Design review of the part built by this model. Coordinates are the model's own, in mm. A direction names the side the tool comes from. Coordinates: 2 decimals unless noted, no trailing zeros. Loops run counter-clockwise (first coordinate to the right, second up) from the corner with the lowest first, then second, coordinate; pieces in that order, holes last. Notation, with made-up numbers: (39, 6.25) -> (61, 6.25) arc R31 ccw to (61, 37.25) -> close; hole circle Ø9 at (14.25, 84). An arc over 180 degrees is marked (long way). Use CSV: the item, a comma, the result in double quotes.
```python
from build123d import *

# Parameters (mm, degrees)
AUFSATZ_LINEAR_AUSTRAGEN1_DEPTH = 2
SKIZZE2_R                       = 1.5
SCHNITT_LINEAR_AUSTRAGEN1_DEPTH = 68.344264789


with BuildPart() as part:
    # Skizze1 → Aufsatz-Linear austragen1 (new body)
    with BuildSketch(Plane.XY):
        Polygon((-50, 17.5), (-50, 7.5), (-50, -2.5), (-50, -7.866530531), (-30, -17.5), (50, -17.5), (50, 17.5), align=None)
        with BuildLine():
            Line((-50, -2.5), (-50, 7.5))
            Line((-50, 7.5), (-60, 7.5))
            ThreePointArc((-60, 7.5), (-56.464466094, 6.035533906), (-55, 2.5))
            ThreePointArc((-55, 2.5), (-56.464466094, -1.035533906), (-60, -2.5))
            Line((-60, -2.5), (-50, -2.5))
        make_face()
        with BuildLine():
            ThreePointArc((-55, 2.5), (-56.464466094, 6.035533906), (-60, 7.5))
            Line((-60, 7.5), (-60, -2.5))
            ThreePointArc((-60, -2.5), (-56.464466094, -1.035533906), (-55, 2.5))
        make_face()
        with BuildLine():
            Line((-60, -2.5), (-60, 7.5))
            ThreePointArc((-60, 7.5), (-64.874594918, 3.612800243), (-62.169780165, -2.004670247))
            ThreePointArc((-62.169780165, -2.004670247), (-61.112800243, -2.374594918), (-60, -2.5))
        make_face()
        with BuildLine():
            Line((-50, -7.866530531), (-50, -2.5))
            Line((-50, -2.5), (-60, -2.5))
            ThreePointArc((-60, -2.5), (-61.112800243, -2.374594918), (-62.169780165, -2.004670247))
            Line((-62.169780165, -2.004670247), (-50, -7.866530531))
        make_face()
    extrude(amount=AUFSATZ_LINEAR_AUSTRAGEN1_DEPTH)

    # Skizze2 → Schnitt-Linear austragen1 (cut, through all)
    with BuildSketch(Plane.XY.offset(2)):
        with Locations((-51.5, 2.5)):
            Circle(SKIZZE2_R)
        with BuildLine():
            Line((-51.5, 4), (-61.5, 4))
            ThreePointArc((-61.5, 4), (-60.439339828, 3.560660172), (-60, 2.5))
            ThreePointArc((-60, 2.5), (-60.439339828, 1.439339828), (-61.5, 1))
            Line((-61.5, 1), (-51.5, 1))
            ThreePointArc((-51.5, 1), (-53, 2.5), (-51.5, 4))
        make_face()
        with Locations((-61.5, 2.5)):
            Circle(SKIZZE2_R)
        with Locations((-25, -7.5)):
            Circle(SKIZZE2_R)
        with Locations((35, -7.5)):
            Circle(SKIZZE2_R)
        with Locations((5, -7.5)):
            Circle(SKIZZE2_R)
    extrude(amount=-SCHNITT_LINEAR_AUSTRAGEN1_DEPTH, mode=Mode.SUBTRACT)


solid = part.part
```
Item 1: Add section C-C (z = 1.35). Give the boundary of the cut face in (x, y).
Checked values:
outline,"(-62.17, -2) -> (-30, -17.5) -> (50, -17.5) -> (50, 17.5) -> (-50, 17.5) -> (-50, 7.5) -> (-60, 7.5) arc R5 ccw to start; hole (-61.5, 1) -> (-51.5, 1) arc R1.5 ccw to (-51.5, 4) -> (-61.5, 4) arc R1.5 ccw to start; hole circle Ø3 at (-25, -7.5); hole circle Ø3 at (5, -7.5); hole circle Ø3 at (35, -7.5)"
Item 2: Machinability: for faces 1 (the face through (-55, 7.5, 1)), 2 (the face through (-50, 2.5, 1)), 3 (the face through (-64.853, 3.704, 0.986)), which of the approach directions +Z, -Z, +X, -X, +Y, -Y give a long, thin tool a straight path to every point of the face, cutting with its end or side? Answer none if there is none.
Checked values:
face 1,"+Z, -Z, -X, +Y"
face 2,"+Z, -Z"
face 3,"+Z, -Z, -X"
Item 3: Clearance check with flat-ended pins moving along their axes: pin 1 (0.6 mm diameter, centred on x = -55, z = 1, fed in from +Y); pin 2 (1 mm diameter, centred on x = -56.5, z = 1, fed in from -Y); pin 3 (4 mm diameter, centred on x = -30, y = -13, fed in from -Z). State where each tip first meets the part, or that it passes through.
Checked values:
pin 1,"y = 7.5"
pin 2,"y = -4.98"
pin 3,"z = 0"
Item 4: Add section A-A (x = 5). Give the boundary of the cut face in (y, z).
Checked values:
outline,"(-17.5, 0) -> (-9, 0) -> (-9, 2) -> (-17.5, 2) -> close; (-6, 0) -> (17.5, 0) -> (17.5, 2) -> (-6, 2) -> close"
Item 5: To check wall thickness, follow line 1 along Y through (x, z) = (-25, 1.1); line 2 along Y through (x, z) = (-58, 1.85); line 3 along X through (y, z) = (9.5, 1.85). State the ranges of each line that lie inside material, in increasing order.
Checked values:
line 1,"-17.5 to -9, -6 to 17.5"
line 2,"-4.01 to 1, 4 to 7.5"
line 3,"-50 to 50"
Item 6: Add section D-D (y = -13). Give the boundary of the cut face in (x, z), then the cut area to 3 significant figures.
Checked values:
outline,"(-39.34, 0) -> (50, 0) -> (50, 2) -> (-39.34, 2) -> close"
area,"179 mm^2"
Item 7: Draft analysis for pull direction X (two halves, no side actions). For faces 4 (the face through (50, 0, 1)), 5 (the face through (-8, 0, 0)), 6 (the face through (-56, 4, 1)), state which applies: pulls with the +X half, pulls with the -X half, needs draft (parallel to the pull), parting line crosses it, or undercut.
Checked values:
face 4,"pulls with the +X half"
face 5,"needs draft"
face 6,"undercut"
Item 8: Add section B-B (y = 2.5). Give the boundary of the cut face in (x, z).
Checked values:
outline,"(-65, 0) -> (-63, 0) -> (-63, 2) -> (-65, 2) -> close; (-50, 0) -> (50, 0) -> (50, 2) -> (-50, 2) -> close"
